Design review of the part built by this model. Coordinates are the model's own, in mm. A direction names the side the tool comes from. Coordinates: 2 decimals unless noted, no trailing zeros. Order: outer loops, then holes, each group sorted by start corner. A loop starts at its lowest first (then second) coordinate and runs counter-clockwise, first axis right, second up. Notation, with made-up numbers: M 85,10 L 138,10 A22 cw 138,19 Z; hole C -33,-29.75 d1. An arc over 180 degrees is marked long. Use CSV: the item, a comma, the result in double quotes.
```python
from build123d import *

# Parameters (mm, degrees)
SKETCH_2_W               = 0.5
SKETCH_2_H               = 1
CUT_EXTRUDE_1_DEPTH      = 0.3
PATTERN_CIRCULAR_1_COUNT = 4


with BuildPart() as part:
    # ｽｹｯﾁ1 → 回転1 (revolve)
    with BuildSketch(Plane.XY, mode=Mode.PRIVATE) as revolve_1_sk:
        Polygon((0, 0), (1.7, 0), (1.7, -0.5), (1, -0.5), (1, -8.5), (0, -8.5), align=None)
    revolve(revolve_1_sk.sketch.rotate(Axis((0, -8.5, 0), (0, 1, 0)), 90), axis=Axis((0, -8.5, 0), (0, 1, 0)))

    # ｽｹｯﾁ2 → ｶｯﾄ - 押し出し1 (cut)
    with BuildSketch(Plane(origin=(0, 0, 0), x_dir=(1, 0, 0), z_dir=(0, 1, 0))):
        with Locations((0, 0.5)):
            Rectangle(SKETCH_2_W, SKETCH_2_H)
    cut_extrude_1 = extrude(amount=-CUT_EXTRUDE_1_DEPTH, mode=Mode.SUBTRACT)

    # 円形ﾊﾟﾀｰﾝ1: ｶｯﾄ - 押し出し1 ×4 about axis
    pattern_circular_1_axis = Axis((0, 0, 0), (0, 1, 0))
    for i in range(1, PATTERN_CIRCULAR_1_COUNT):
        add(cut_extrude_1.rotate(pattern_circular_1_axis, i * 360 / PATTERN_CIRCULAR_1_COUNT), mode=Mode.SUBTRACT)


solid = part.part
```
(1) Wall thickness on probe 1 along Y at (x, z) = (-0.05, -1.3); probe 2 along Y at (x, z) = (-0.1, -0.05); probe 3 along X at (y, z) = (-2, -0.45): over which ranges is each line inside the solid? List them lowest first.
The answers:
probe 1,"y = -0.5 to 0"
probe 2,"y = -8.5 to -0.3"
probe 3,"x = -0.89 to 0.89"
(2) Add section D-D on z = -1.15. State the section outline as (x, y) points.
The answers:
outline,"M -1.25,-0.5 L 1.25,-0.5 L 1.25,0 L -1.25,0 Z"
(3) Clearance check with flat-ended pins moving along their axes: P1, Ø1, axis at y = -4, z = 0.5, coming from the +X side; P2, Ø1.5, axis at y = -7.5, z = 0, coming from the -X side; P3, Ø1, axis at x = -0.5, y = -3.5, coming from the +Z side. State where each tip first meets the part, or that it passes through.
The answers:
P1,"stops at x = 1"
P2,"stops at x = -1"
P3,"stops at z = 1"
(4) The part is to be moulded in two halves that separate along Z. For faces 1 (the face through (1, -5, 0)), 2 (the face through (0, -0.3, 0)), 3 (the face through (0, -8.5, 0)), say which applies: pulls with the +Z half, pulls with the -Z half, needs draft (parallel to the pull), parting line crosses it, or undercut.
The answers:
face 1,"parting line crosses it"
face 2,"undercut"
face 3,"needs draft"
(5) Add section A-A on z = 0. State the section outline as (x, y) points.
The answers:
outline,"M -1.7,-0.5 L -1,-0.5 L -1,-8.5 L 1,-8.5 L 1,-0.5 L 1.7,-0.5 L 1.7,0 L 1,0 L 1,-0.3 L -1,-0.3 L -1,0 L -1.7,0 Z"
(6) Add section B-B on x = 0. State the section outline as (y, z) points, and give its area (3 significant figures).
The answers:
outline,"M -8.5,-1 L -0.5,-1 L -0.5,-1.7 L 0,-1.7 L 0,-1 L -0.3,-1 L -0.3,1 L 0,1 L 0,1.7 L -0.5,1.7 L -0.5,1 L -8.5,1 Z"
area,"17.1 mm2"
(7) For faces 4 (the face through (1, -0.5, -1)), 5 (the face through (0.4, 0, -0.4)), list the 3-axis set-ups (+Z, -Z, +X, -X, +Y, -Y) from which the entire face can be reached by the end or side of a thin tool; tool diameter is ignored.
The answers:
face 4,"-Y"
face 5,"+Z, -Z, +X, -X, +Y"
(8) Add section C-C on y = -5.25. State the section outline as (x, z) points, and give its area (3 significant figures).
The answers:
outline,"C 0,0 d2"
area,"3.14 mm2"
